Job drawing, mm, ordinate dimensions from the low corner. One solid piece. Give positions to 0.01 mm unless a question says otherwise; leave off trailing zeros. Order: outer loops, then holes, each group sorted by start corner. A loop starts at its lowest first (then second) coordinate and runs counter-clockwise, first axis right, second up. Notation, with made-up numbers: (-16.75, 39) - (1.25, 39) arc R29 cw to (1.25, 59) - close; hole circle Ø9 at (28.25, 60.5). An arc over 180 degrees is marked (long way). Write each question's results on one line, items separated by ' | '. Start each with the question number.
1) Cut at B-B on z = 40. List the corners of the cut face in (x, y).
2) Drill centre lines: line 1 along Y through (x, z) = (50, 73.5); line 2 along X through (y, z) = (3, 16.5); line 3 along X through (y, z) = (80, 45.5). Where is each one in solid material? Low to high. Write a range as from..to.
3) Cut at D-D on z = 63.5. List the corners of the cut face in (x, y).
4) Drop flat-ended pins along their axis: pin 1 Ø3 at (x, y) = (62, 38.5) entering from +Z; pin 2 Ø1 at (y, z) = (66.5, 51) entering from -X; pin 3 Ø5 at (x, z) = (60, 26.5) entering from +Y. Give the stop position or say it passes through.
5) Cut at A-A on x = 40. List the corners of the cut face in (y, z).
6) Cut at C-C on y = 20. List the corners of the cut face in (x, z).
7) Two-plate mould, pull along X, no slides. Class the marked faces 1 and 2: +X half, -X half, draft (parallel to the pull), parting line (faces both ways), or undercut.
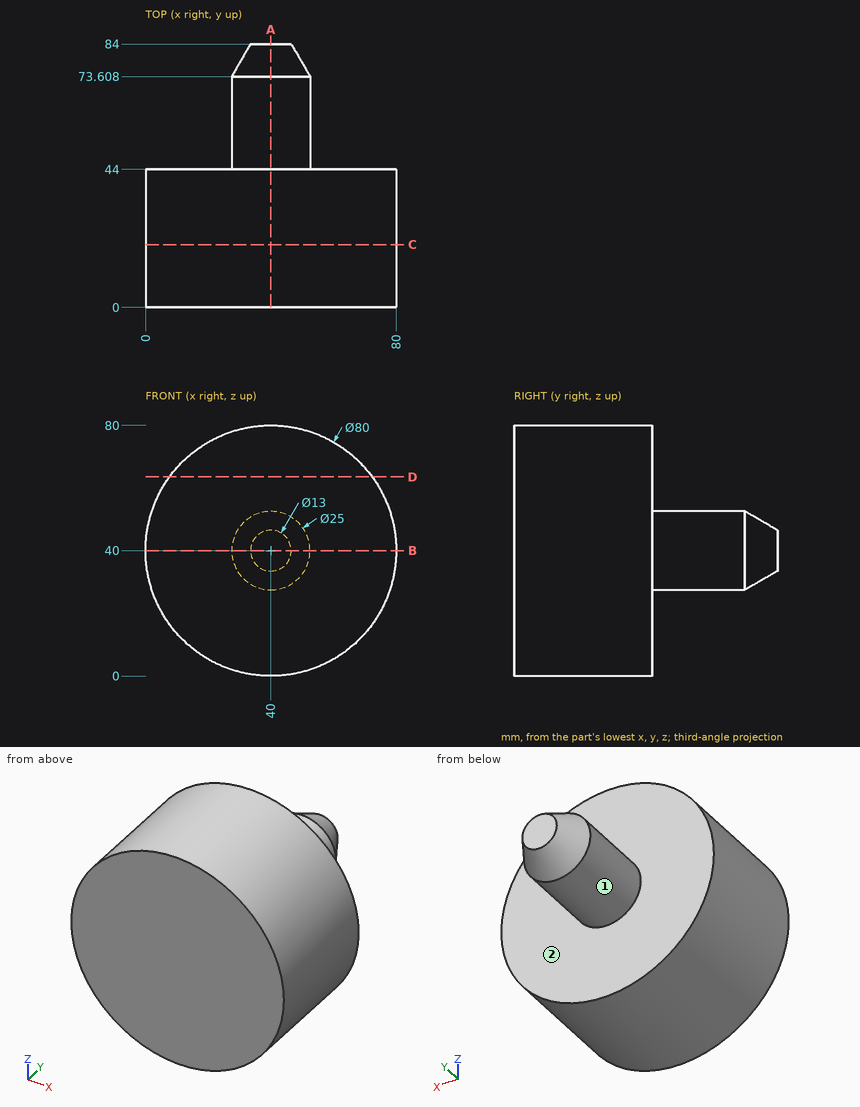
Results:
1) outline: (0, 0) - (80, 0) - (80, 44) - (52.5, 44) - (52.5, 73.61) - (46.5, 84) - (33.5, 84) - (27.5, 73.61) - (27.5, 44) - (0, 44) - close
2) line 1: 0..44 | line 2: 7.63..72.37 | line 3: 33.12..46.88
3) outline: (7.63, 0) - (72.37, 0) - (72.37, 44) - (7.63, 44) - close
4) pin 1: z = 74.35 | pin 2: x = 33.22 | pin 3: y = 44
5) outline: (0, 0) - (44, 0) - (44, 27.5) - (73.61, 27.5) - (84, 33.5) - (84, 46.5) - (73.61, 52.5) - (44, 52.5) - (44, 80) - (0, 80) - close
6) outline: circle Ø80 at (40, 40)
7) face 1: parting line | face 2: draft
